The drawing under review shows one solid part. Ordinate dimensions are in mm from its lowest x, y, z. Give positions to 0.01 mm unless a question says otherwise; leave off trailing zeros. Order: outer loops, then holes, each group sorted by start corner. A loop starts at its lowest first (then second) coordinate and runs counter-clockwise, first axis right, second up. Notation, with made-up numbers: (20, 78) - (46, 78) arc R23 ccw to (46, 98) - close; hole circle Ø5 at (-34.75, 28). An arc over 180 degrees is marked (long way). Use CSV: the item, a comma, the result in double quotes. Start each with the question number.
1. Draft analysis for pull direction X (two halves, no side actions). For the marked faces 1 and 2, state which applies: released by +X, released by -X, zero draft, split by the parting line, or undercut.
2. To check wall thickness, follow line 1 (X direction, y = 32, z = 52); line 2 (X direction, y = 26, z = 28); line 3 (Z direction, x = 123.5, y = 56). State the ranges of each line that lie inside material, in increasing order. Write a range as [from, to].
3. Take a section at C-C, the plane y = 42. State the section outline as (x, z) points.
4. Take a section at A-A, the plane z = 11. State the section outline as (x, y) points.
5. Take a section at B-B, the plane x = 43. State the section outline as (y, z) points, then the cut area to 3 significant figures.
6. For pin 1 (3 mm diameter, centred on x = 15, z = 46.5, fed in from -Y); pin 2 (10 mm diameter, centred on x = 18, z = 38, fed in from -Y); pin 3 (1.5 mm diameter, centred on x = 23.5, z = 31.5, fed in from +Y), all flat-tipped, find the tip position at first contact; note any pin that passes through.
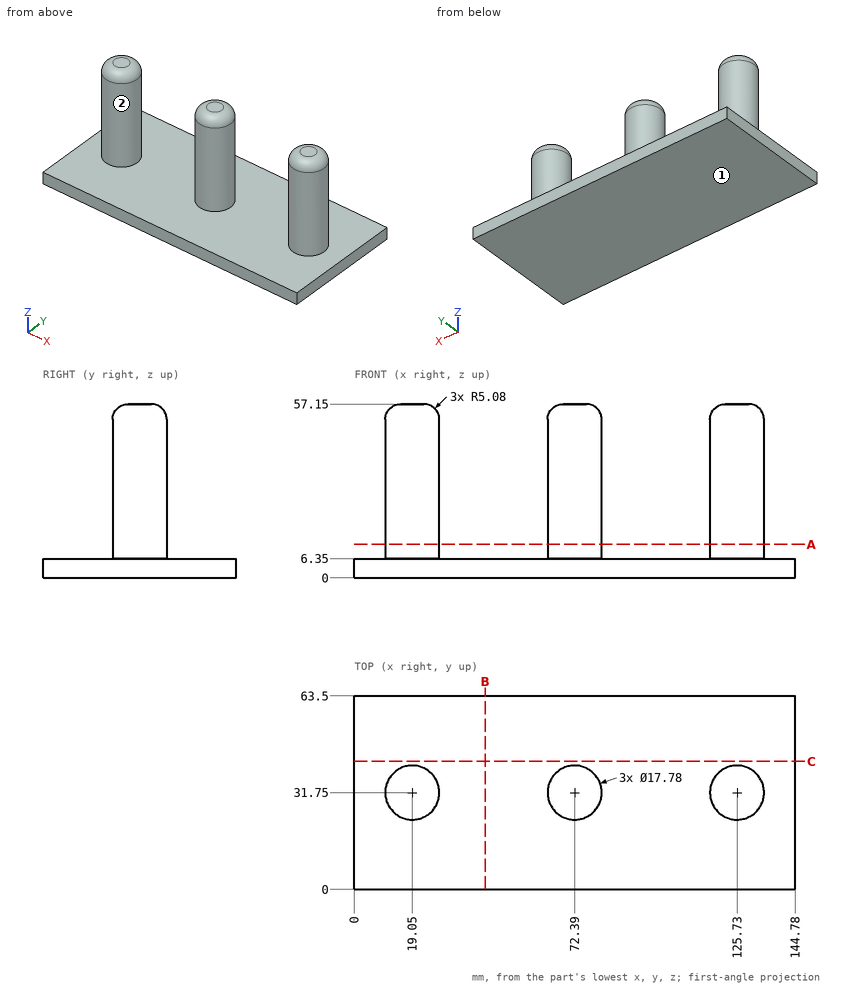
Determined:
1,face 1,"zero draft"
1,face 2,"undercut"
2,line 1,"x = [10.16, 27.94], [63.5, 81.28], [116.84, 134.62]"
2,line 2,"x = [12.27, 25.83], [65.61, 79.17], [118.95, 132.51]"
2,line 3,"z = [0, 6.35]"
3,outline,"(0, 0) - (144.78, 0) - (144.78, 6.35) - (0, 6.35) - close"
4,outline,"circle Ø17.78 at (19.05, 31.75); circle Ø17.78 at (72.39, 31.75); circle Ø17.78 at (125.73, 31.75)"
5,outline,"(0, 0) - (63.5, 0) - (63.5, 6.35) - (0, 6.35) - close"
5,area,"403 mm²"
6,pin 1,"stops at y = 23.23"
6,pin 2,"stops at y = 22.86"
6,pin 3,"stops at y = 39.83"
